Drawing for the job (mm, zero at the part's lowest x, y, z). A direction names the side the tool comes from. Coordinates: 2 decimals unless noted, no trailing zeros. Write each loop counter-clockwise with the first axis right and the second up, starting at its lowest first coordinate (ties: lowest second). Pieces come first, ordered by that corner, then holes. Notation, with made-up numbers: (-0.75, -24) -> (55.25, -24) arc R8 cw to (55.25, -9) -> close; hole circle Ø7 at (3, 73). An arc over 180 degrees is marked (long way). Write item = value, one per line. Start each with the question number.
Q1. Probe line 1 (Y direction, x = 21.5, z = 8.75); line 2 (Z direction, x = 16.5, y = 6); line 3 (X direction, y = 29, z = 4.5). List the from-to ranges inside material, lowest first.
Q2. Band-saw the part on C-C, the plane z = 13.5. List the corners of the cut face in (x, y), plus the area to 3 significant figures.
Q3. Pull direction Y, two halves, no side cores. Call the marked faces 4, 5 and 6: released by +Y, released by -Y, zero draft, split by the parting line, or undercut.
Q4. Tool access for the marked faces 1, 2 and 3: list every direction of +Z, -Z, +X, -X, +Y, -Y with a clear straight run to the whole face (end or side of a thin tool).
Q5. Band-saw the part on A-A, the plane x = 21.5. List the corners of the cut face in (y, z).
Q6. Band-saw the part on D-D, the plane y = 5. List the corners of the cut face in (x, z), plus the area to 3 significant figures.
Q7. Pin check, flat tips, straight feed: P1, Ø1.5, axis at x = 22.5, z = 3, coming from the +Y side; P2, Ø12, axis at y = 14.5, z = 3.5, coming from the -X side; P3, Ø4, axis at y = 19, z = 20, coming from the -X side. Stop position of each tip, or through.
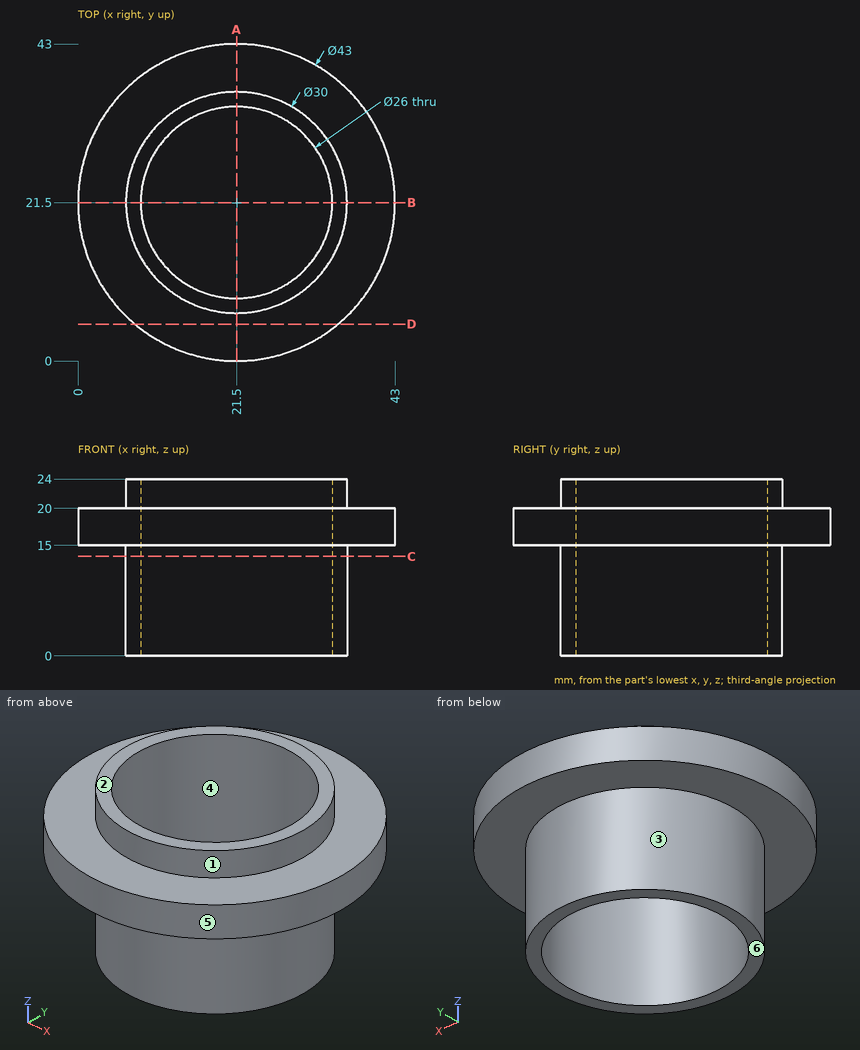
Ans:
q1.line_1 = 6.5 to 8.5, 34.5 to 36.5
q1.line_2 = 15 to 20
q1.line_3 = 8.51 to 10.88, 32.12 to 34.49
q2.outline = circle Ø30 at (21.5, 21.5); hole circle Ø26 at (21.5, 21.5)
q2.area = 176 mm2
q3.face_4 = undercut
q3.face_5 = split by the parting line
q3.face_6 = zero draft
q4.face_1 = +Z
q4.face_2 = +Z, +X, -X, +Y, -Y
q4.face_3 = -Z
q5.outline = (0, 15) -> (6.5, 15) -> (6.5, 0) -> (8.5, 0) -> (8.5, 24) -> (6.5, 24) -> (6.5, 20) -> (0, 20) -> close; (34.5, 0) -> (36.5, 0) -> (36.5, 15) -> (43, 15) -> (43, 20) -> (36.5, 20) -> (36.5, 24) -> (34.5, 24) -> close
q6.outline = (7.72, 15) -> (35.28, 15) -> (35.28, 20) -> (7.72, 20) -> close
q6.area = 138 mm2
q7.P1 = 36.5
q7.P2 = 6.53
q7.P3 = 0.01
